Source: CAD feature listing. Evaluate the final solid. Frame: model axes, mm. A direction names the side the tool comes from. Round coordinates to 2 decimals unless told otherwise and drop trailing zeros. Order: outer loops, then holes, each group sorted by start corner. A loop starts at its lowest first (then second) coordinate and runs counter-clockwise, first axis right, second up. Notation, with made-up numbers: M 0,-32 L 16,-32 A26 ccw 16,-4 Z; hole C 16.25,-38 d10. An arc over 180 degrees is marked long. Answer as CSV lines item,"result". Start each with the question number.
Item 1: First-contact query: P1, Ø2.5, axis at x = -8.49, y = 8.49, coming from the +Z side; P2, Ø4, axis at x = 4.5, y = -11.5, coming from the +Z side; P3, Ø1.5, axis at y = 5.5, z = -4.5, coming from the -X side; P4, Ø8, axis at y = -10, z = -20.5, coming from the +X side. Flat tips, straight axial feed; report the tip coordinate or a pass-through.
Item 2: Section query A-A on x = 0. Return the cut outline in (y, z).
Item 3: Section query C-C on z = -1. Return the cut outline in (x, y), plus the area to 3 significant figures.
Item 4: Pull-direction query (X, two-part tool) for faces 1 (the face through (-7.68, 9.75, -13.31)), 2 (the face through (7, -7, -27)), 3 (the face through (-6.633, -6.083, -28.479)); classes: +X half, -X half, draft (parallel to the pull), parting line (faces both ways), or undercut.
Item 5: Set-up query: faces 4 (the face through (-1.172, 8.923, 0.986)), 5 (the face through (9.29, -9.75, -13.31)). Return all of +Z, -Z, +X, -X, +Y, -Y with unobstructed straight access to the full face (end or side cutting, diameter ignored); none if empty.
Item 6: Section query D-D on y = 13.5. Return the cut outline in (x, z), plus the area to 3 significant figures.
Item 7: Line query: line 1 (Y direction, x = -8.5, z = -1.5); line 2 (X direction, y = 8, z = -16); line 3 (Z direction, x = 2.5, y = 11). Output: solid intervals per line, ascending. Write a range as [from, to].
from build123d import *

# Parameters (mm, degrees)
ESQUISSE3_R             = 16
ESQUISSE3_R_2           = 9
BOSS_EXTRU_1_DEPTH      = 27
ESQUISSE3_3_R           = 9
ESQUISSE3_3_R_2         = 7.5
BOSS_EXTRU_2_DEPTH      = 2
ESQUISSE7_R             = 9
ESQUISSE7_R_2           = 7.5
BOSS_EXTRU_3_DEPTH      = 30
ESQUISSE8_R             = 1.5
ENL_V_MAT_EXTRU_1_DEPTH = 30


with BuildPart() as part:
    # Esquisse3 → Boss.-Extru.1 (new body)
    with BuildSketch(Plane.XY):
        Circle(ESQUISSE3_R)
        Circle(ESQUISSE3_R_2, mode=Mode.SUBTRACT)
    extrude(amount=-BOSS_EXTRU_1_DEPTH)



with BuildPart() as body_2:
    # Esquisse3_3 → Boss.-Extru.2 (new body)
    with BuildSketch(Plane.XY):
        Circle(ESQUISSE3_3_R)
        Circle(ESQUISSE3_3_R_2, mode=Mode.SUBTRACT)
    extrude(amount=BOSS_EXTRU_2_DEPTH)


with BuildPart() as part_1:
    add(part.part)

    add(body_2.part)  # Boss.-Extru.3 merges body 2
    # Esquisse7 → Boss.-Extru.3 (add)
    with BuildSketch(Plane(origin=(0, 0, 0), x_dir=(-1, 0, 0), z_dir=(0, 0, -1))):
        with Locations(Location((0, 0, 0), (0, 0, 180))):
            Circle(ESQUISSE7_R)
        with Locations(Location((0, 0, 0), (0, 0, 180))):
            Circle(ESQUISSE7_R_2, mode=Mode.SUBTRACT)
    extrude(amount=BOSS_EXTRU_3_DEPTH)

    # Esquisse8 → Enl_v. mat.-Extru.1 (cut)
    with BuildSketch(Plane.XY):
        with Locations((-8.485281374, 8.485281374)):
            Circle(ESQUISSE8_R)
        with Locations((8.485281374, 8.485281374)):
            Circle(ESQUISSE8_R)
    enl_v_mat_extru_1 = extrude(amount=-ENL_V_MAT_EXTRU_1_DEPTH, mode=Mode.SUBTRACT)

    # Sym_trie1: Enl_v. mat.-Extru.1 across plane
    add(enl_v_mat_extru_1.mirror(Plane.ZX), mode=Mode.SUBTRACT)


solid = part_1.part
Results:
1,P1,"through"
1,P2,"z = 0"
1,P3,"x = -15.28"
1,P4,"x = 14.83"
2,outline,"M -16,-27 L -9,-27 L -9,-30 L -7.5,-30 L -7.5,2 L -9,2 L -9,0 L -16,0 Z; M 7.5,-30 L 9,-30 L 9,-27 L 16,-27 L 16,0 L 9,0 L 9,2 L 7.5,2 Z"
3,outline,"C 0,0 d32; hole C -8.49,-8.49 d3; hole C -8.49,8.49 d3; hole C 0,0 d15; hole C 8.49,-8.49 d3; hole C 8.49,8.49 d3"
3,area,"599 mm^2"
4,face 1,"undercut"
4,face 2,"draft"
4,face 3,"parting line"
5,face 4,"+Z"
5,face 5,"+Z, -Z"
6,outline,"M -8.59,-27 L 8.59,-27 L 8.59,0 L -8.59,0 Z"
6,area,"464 mm^2"
7,line 1,"[-13.56, -9.99], [-6.99, 6.99], [9.99, 13.56]"
7,line 2,"[-13.86, -9.9], [-7.07, 7.07], [9.9, 13.86]"
7,line 3,"[-27, 0]"
